Input: part model. Units: mm. Frame: model coordinates. Face numbers are marked on the shaded views. Give positions to 0.01 mm unless a question says otherwise; leave off trailing zeros. Order: outer loops, then holes, each group sorted by start corner. A loop starts at its lowest first (then second) coordinate and runs counter-clockwise, first axis right, second up. Notation, with made-up numbers: (66, -14) - (81, -14) arc R18 cw to (81, 20) - close; hole circle Ø6 at (88, -3). An arc over 180 degrees is marked (long way). Answer in a Markdown table with one row per item. Add a question column.
1. Mould query, pull axis X, two halves, no side actions, for the marked faces 1, 2 and 3. Classes: released by +X, released by -X, zero draft, split by the parting line, or undercut.
2. Section query D-D on x = 46. Return loops of the section in (y, z).
3. Section query A-A on y = -160. Return loops of the section in (x, z).
4. Contact query for flat-ended pins moving along their axis: pin 1 (1 mm diameter, centred on y = -112.5, z = 28, fed in from +X); pin 2 (1.5 mm diameter, centred on x = 20.5, y = -114, fed in from +Z); pin 3 (4.5 mm diameter, centred on y = -130, z = 15, fed in from -X). Output: stop coordinate, or through.
5. Ray query, line 1 (Y direction, x = 2.8, z = 32); line 2 (Y direction, x = 2.75, z = 15); line 3 (X direction, y = 190, z = 2.1). Return the intervals inside material, ascending. Write a range as [from, to].
6. Section query B-B on y = 15.5. Return loops of the section in (x, z).
7. Section query C-C on z = 47. Return loops of the section in (x, y).
```python
from build123d import *

# Parameters (mm, degrees)
PAD_DEPTH         = 200
SKETCH001_R       = 2.5
POCKET_DEPTH      = 4.001
POCKET_DEPTH_BACK = -47.001
SKETCH003_R       = 2.5
SKETCH003_R_2     = 6.5
POCKET001_DEPTH   = 51.001


with BuildPart() as part:
    # Sketch → Pad (new body, symmetric)
    with BuildSketch(Plane.XZ):
        Polygon((0, 51), (0, 0), (51, 0), (51, 4), (4, 4), (4, 51), align=None)
    extrude(amount=PAD_DEPTH, both=True)

    # Sketch001 → Pocket (cut, two sides)
    with BuildSketch(Plane(origin=(0, 0, 4), x_dir=(-1, 0, 0), z_dir=(0, 0, 1))) as pocket_sk:
        with Locations((-26.435764, 190)):
            Circle(SKETCH001_R)
        with Locations((-26.435764, -190)):
            Circle(SKETCH001_R)
    extrude(amount=-POCKET_DEPTH, mode=Mode.SUBTRACT)
    extrude(pocket_sk.sketch, amount=-POCKET_DEPTH_BACK, mode=Mode.SUBTRACT)

    # Sketch003 → Pocket001 (cut, through all)
    with BuildSketch(Plane(origin=(0, 0, 0), x_dir=(0, 0, -1), z_dir=(-1, 0, 0))):
        with Locations((-15, 130)):
            Circle(SKETCH003_R)
        with Locations((-15, -130)):
            Circle(SKETCH003_R)
        with Locations((-15, -30)):
            Circle(SKETCH003_R)
        with Locations((-15, 24)):
            Circle(SKETCH003_R)
        with Locations((-32, 160)):
            Circle(SKETCH003_R_2)
        with Locations((-32, 192)):
            Circle(SKETCH003_R)
        with Locations((-32, 128)):
            Circle(SKETCH003_R)
    extrude(amount=-POCKET001_DEPTH, mode=Mode.SUBTRACT)


solid = part.part
```
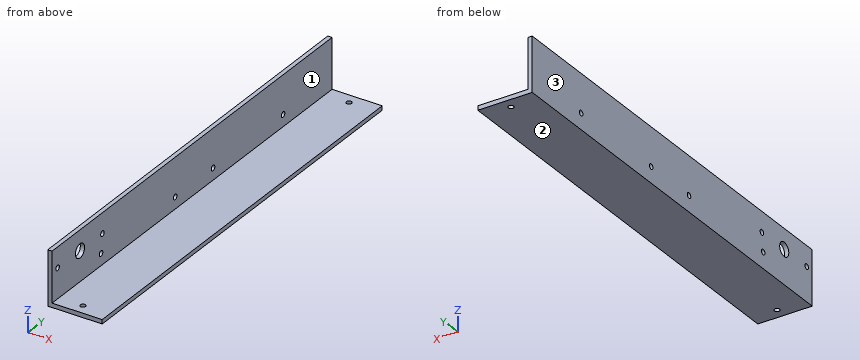
Answer:
| question | item | result |
|---|---|---|
| 1 | face 1 | released by +X |
| 1 | face 2 | zero draft |
| 1 | face 3 | released by -X |
| 2 | outline | (-200, 0) - (200, 0) - (200, 4) - (-200, 4) - close |
| 3 | outline | (0, 0) - (51, 0) - (51, 4) - (4, 4) - (4, 25.5) - (0, 25.5) - close; (0, 38.5) - (4, 38.5) - (4, 51) - (0, 51) - close |
| 4 | pin 1 | stops at x = 4 |
| 4 | pin 2 | stops at z = 4 |
| 4 | pin 3 | passes through |
| 5 | line 1 | y = [-200, -194.5], [-189.5, -166.5], [-153.5, -130.5], [-125.5, 200] |
| 5 | line 2 | y = [-200, -132.5], [-127.5, -26.5], [-21.5, 27.5], [32.5, 127.5], [132.5, 200] |
| 5 | line 3 | x = [0, 23.94], [28.94, 51] |
| 6 | outline | (0, 0) - (51, 0) - (51, 4) - (4, 4) - (4, 51) - (0, 51) - close |
| 7 | outline | (0, -200) - (4, -200) - (4, 200) - (0, 200) - close |
